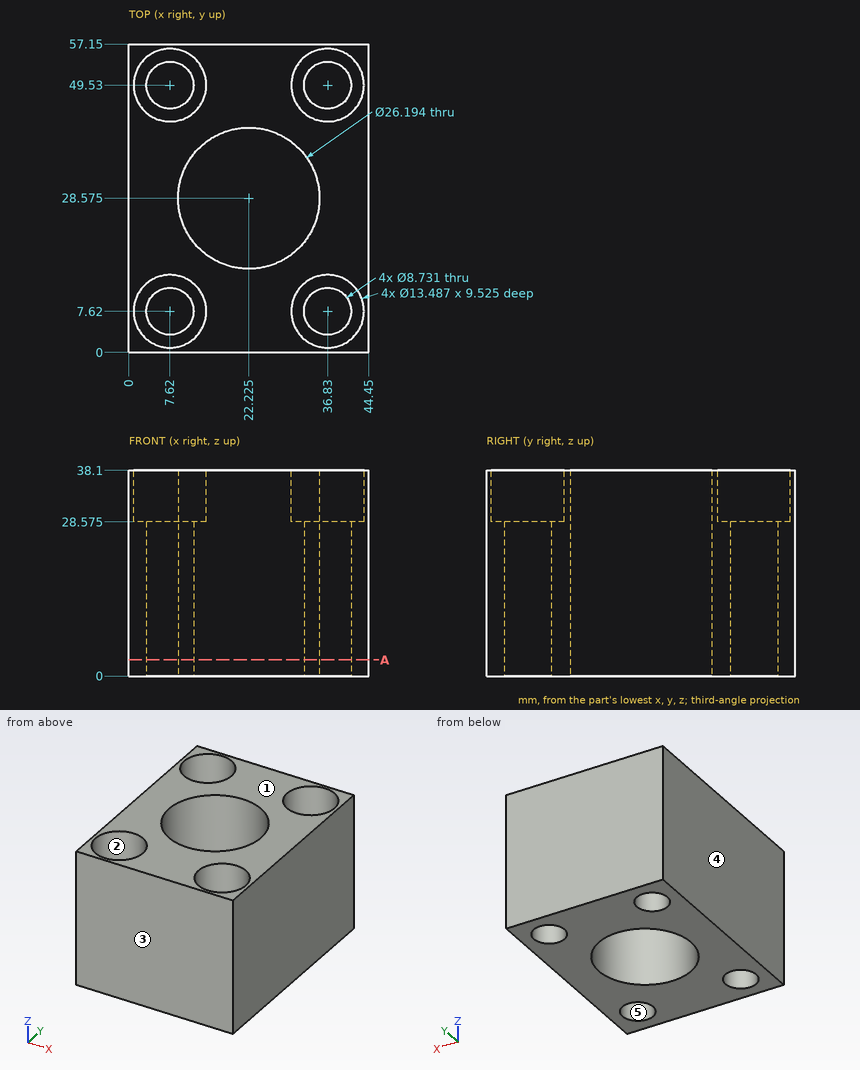
Part print with two shaded views. Sizes in mm from the minimum x, y, z corner. A direction names the side the tool comes from. Give positions to 0.01 mm unless a question says otherwise; leave off trailing zeros. Put each result on its own line as item: value.
Q1. Mould opens along Y. For the marked faces 3, 4 and 5 say: pulls with the +Y half, pulls with the -Y half, needs draft (parallel to the pull), parting line crosses it, or undercut.
Filled in:
face 3: pulls with the -Y half
face 4: needs draft
face 5: undercut
Q2. Slice it at A-A (z = 3). Give the number of separate pieces and of enclosed holes in the cut face, plus the area to 3 significant figures.
Filled in:
separate pieces: 1
enclosed holes: 5
area: 1,760 mm²
Q3. Flat gauge pins, fed straight in: pin 1 (8 mm diameter, centred on x = 36.83, y = 49.53, fed in from +Z); pin 2 (6.5 mm diameter, centred on x = 39.5, y = 5.5, fed in from +Z) (3 decimals). Where does each tip first touch, or does it go through?
Filled in:
pin 1: passes through
pin 2: stops at z = 28.575
Q4. Tool access for the marked faces 1 and 2: list every direction of +Z, -Z, +X, -X, +Y, -Y with a clear straight run to the whole face (end or side of a thin tool).
Filled in:
face 1: +Z, +X, -X, +Y, -Y
face 2: +Z
Q5. Probe line 1 along Y through (x, z) = (36.83, 33); line 2 along X through (y, z) = (8, 7.5); line 3 along Y through (x, z) = (36, 33). List the from-to ranges inside material, lowest first.
Filled in:
line 1: y = 0 to 0.88, 14.36 to 42.79, 56.27 to 57.15
line 2: x = 0 to 3.27, 11.97 to 32.48, 41.18 to 44.45
line 3: y = 0 to 0.93, 14.31 to 42.84, 56.22 to 57.15
